from build123d import *

# Parameters (mm, degrees)
SKETCH1_R           = 2.5
BOSS_EXTRUDE1_DEPTH = 5


with BuildPart() as part:
    # Sketch1 → Boss-Extrude1 (new body)
    with BuildSketch(Plane.XY):
        Polygon((-49.999307958, 92.545526446), (60.000692042, 92.545526446), (60.000692042, -57.454473554), (-49.999307958, -57.454473554), (-49.999307958, -130.954473554), (-49.999307958, -160.954473554), (-149.999307958, -160.954473554), (-149.999307958, -130.954473554), (-69.999307958, -130.954473554), (-69.999307958, 166.045526446), (-149.999307958, 166.045526446), (-149.999307958, 196.045526446), (-49.999307958, 196.045526446), (-49.999307958, 166.045526446), align=None)
        with Locations((-34.999307958, 17.545526446)):
            Circle(SKETCH1_R, mode=Mode.SUBTRACT)
        with Locations((30.000692042, -47.454473554)):
            Circle(SKETCH1_R, mode=Mode.SUBTRACT)
        with Locations((30.000692042, 82.545526446)):
            Circle(SKETCH1_R, mode=Mode.SUBTRACT)
    extrude(amount=BOSS_EXTRUDE1_DEPTH)


solid = part.part
Check sheet for the modelled part. Datum: model origin and axes. Units: mm. Coordinates: 2 decimals unless noted, no trailing zeros. Loops run counter-clockwise (first coordinate to the right, second up) from the corner with the lowest first, then second, coordinate; pieces in that order, holes last. Notation, with made-up numbers: (-35, -18.5) -> (-16, -18.5) arc R16 cw to (-16, 11.5) -> close; hole circle Ø11 at (6.25, 89.5). An arc over 180 degrees is marked (long way). Write item = value, one per line. Start each with the question number.
1. Section check D-D on x = -25. Record the cut outline in (y, z).
2. Section check B-B on z = 4. Record the cut outline in (x, y).
3. Section check C-C on y = 52. Record the cut outline in (x, z).
4. Depth check by flat-ended pin: P1, Ø1.5, axis at y = 142, z = 2, coming from the +X side; P2, Ø2.5, axis at y = -54, z = 2, coming from the -X side; P3, Ø8, axis at x = 30, y = 82.55, coming from the -Z side; P4, Ø1.5, axis at x = 0.5, z = 3, coming from the +Y side. Enter the tip coordinate at first touch or a pass-through.
5. Section check A-A on x = -131.5. Record the cut outline in (y, z), then the cut area to 3 significant figures.
6. Material ranges on line 1 (X direction, y = -143, z = 0.8); line 2 (Y direction, x = -136.5, z = 4.7); line 3 (X direction, y = 97, z = 4), recorded low to high.
Responses:
q1.outline = (-57.45, 0) -> (92.55, 0) -> (92.55, 5) -> (-57.45, 5) -> close
q2.outline = (-150, -160.95) -> (-50, -160.95) -> (-50, -57.45) -> (60, -57.45) -> (60, 92.55) -> (-50, 92.55) -> (-50, 196.05) -> (-150, 196.05) -> (-150, 166.05) -> (-70, 166.05) -> (-70, -130.95) -> (-150, -130.95) -> close; hole circle Ø5 at (-35, 17.55); hole circle Ø5 at (30, -47.45); hole circle Ø5 at (30, 82.55)
q3.outline = (-70, 0) -> (60, 0) -> (60, 5) -> (-70, 5) -> close
q4.P1 = -50
q4.P2 = -70
q4.P3 = 0
q4.P4 = 92.55
q5.outline = (-160.95, 0) -> (-130.95, 0) -> (-130.95, 5) -> (-160.95, 5) -> close; (166.05, 0) -> (196.05, 0) -> (196.05, 5) -> (166.05, 5) -> close
q5.area = 300 mm2
q6.line_1 = -150 to -50
q6.line_2 = -160.95 to -130.95, 166.05 to 196.05
q6.line_3 = -70 to -50
